from build123d import *

# Parameters (mm, degrees)
SKETCH005_R  = 42.5
PAD005_DEPTH = 85
FILLET_R     = 4
FILLET001_R  = 3
SKETCH006_R  = 16
PAD006_DEPTH = 8
SKETCH007_R  = 4
PAD007_DEPTH = 30
SKETCH008_R  = 2.5
PAD008_DEPTH = 10
PAD009_DEPTH = 7
SKETCH010_R  = 16
PAD010_DEPTH = 10


with BuildPart() as part:
    # Sketch005 → Pad005 (new body)
    with BuildSketch(Plane.XZ):
        Circle(SKETCH005_R)
    extrude(amount=-PAD005_DEPTH)

    # Fillet
    fillet_edges = [part.edges().sort_by_distance(p)[0] for p in [
        (-42.5, 0, 0),
    ]]
    fillet(fillet_edges, radius=FILLET_R)

    # Fillet001
    fillet001_edges = [part.edges().sort_by_distance(p)[0] for p in [
        (-42.5, 85, 0),
    ]]
    fillet(fillet001_edges, radius=FILLET001_R)

    # Sketch006 (on Face5 of Fillet001) → Pad006 (new body)
    with BuildSketch(Plane.XZ):
        Circle(SKETCH006_R)
    extrude(amount=PAD006_DEPTH)

    # Sketch007 (on Face7 of Pad006) → Pad007 (new body)
    with BuildSketch(Plane.XZ.offset(8)):
        Circle(SKETCH007_R)
    extrude(amount=PAD007_DEPTH)

    # Sketch008 (on Face5 of Pad007) → Pad008 (new body)
    with BuildSketch(Plane.XZ):
        with Locations((-35, 0)):
            Circle(SKETCH008_R)
        with Locations((35, 0)):
            Circle(SKETCH008_R)
    extrude(amount=PAD008_DEPTH)

    # Sketch009 (on Face4 of Pad008) → Pad009 (new body)
    with BuildSketch(Plane(origin=(0, 85, 0), x_dir=(1, 0, 0), z_dir=(0, 1, 0))):
        with BuildLine():
            Line((-20.512191, 20.5), (20.512191, 20.5))
            ThreePointArc((20.512191, -20.5), (29, 0), (20.512191, 20.5))
            Line((-20.512191, -20.5), (20.512191, -20.5))
            ThreePointArc((-20.512191, 20.5), (-29, 0), (-20.512191, -20.5))
        make_face()
    extrude(amount=PAD009_DEPTH)

    # Sketch010 (on Face13 of Pad009) → Pad010 (new body)
    with BuildSketch(Plane(origin=(0, 92, 0), x_dir=(1, 0, 0), z_dir=(0, 1, 0))):
        Circle(SKETCH010_R)
    extrude(amount=PAD010_DEPTH)


solid = part.part
Can you work these out from the model? Positions are in its coordinate system, mm. A direction names the side the tool comes from. Coordinates: 2 decimals unless noted, no trailing zeros. Order: outer loops, then holes, each group sorted by start corner. A loop starts at its lowest first (then second) coordinate and runs counter-clockwise, first axis right, second up. Notation, with made-up numbers: M 8.25,68 L 55.25,68 A17 cw 55.25,99 Z; hole C -2,-37.75 d10. An arc over 180 degrees is marked long. Answer as CSV lines item,"result".
(1) On a 3-axis mill with a long thin cutter (end or side, diameter ignored), from which of +Z, -Z, +X, -X, +Y, -Y can I reach the whole of each face in a straight line? I mean faces 1 (the flat face through (13.3, 92, -9.4)), 2 (the flat face through (3, -8, -3)), 3 (the flat face through (35, -10, 0)), 4 (the flat face through (0, 88, 20.5)). Say none if no direction works.
Geometry check:
face 1,"+Y"
face 2,"-Y"
face 3,"+Z, -Z, +X, -Y"
face 4,"+Z, +X, -X, +Y"
(2) I'm going to push flat-ended pins straight in: pin 1 (5 mm diameter, centred on x = 7, z = -32, fed in from -Y); pin 2 (5.5 mm diameter, centred on x = 35.5, z = 0, fed in from -Y); pin 3 (3.5 mm diameter, centred on x = 7.5, y = 90, fed in from +Z). Where does each tip first touch, or does it pass through?
Geometry check:
pin 1,"y = 0"
pin 2,"y = -10"
pin 3,"z = 20.5"
(3) Suppose I cut it at C-C on y = 53.5. Please give me the cut outline in (x, z), plus the area to 3 significant figures.
Geometry check:
outline,"C 0,0 d85"
area,"5,670 mm^2"
(4) Suppose I cut it at B-B on x = 0. Please give me the cut outline in (y, z).
Geometry check:
outline,"M -38,-4 L -8,-4 L -8,-16 L 0,-16 L 0,-38.5 A4 ccw 4,-42.5 L 82,-42.5 A3 ccw 85,-39.5 L 85,-20.5 L 92,-20.5 L 92,-16 L 102,-16 L 102,16 L 92,16 L 92,20.5 L 85,20.5 L 85,39.5 A3 ccw 82,42.5 L 4,42.5 A4 ccw 0,38.5 L 0,16 L -8,16 L -8,4 L -38,4 Z"
(5) Please list where these lines run through material, in increasing order: L1, parallel to Y at x = -6.5, z = -28.5; L2, parallel to Y at x = -19.5, z = 15.5; L3, parallel to X at y = -27.5, z = 0.5.
Geometry check:
L1,"0 to 85"
L2,"0 to 92"
L3,"-3.97 to 3.97"
